Check sheet for the modelled part. Datum: model origin and axes. Units: mm. Face numbers are marked on the shaded views. A direction names the side the tool comes from. Give positions to 0.01 mm unless a question says otherwise; leave off trailing zeros. Loops run counter-clockwise (first coordinate to the right, second up) from the corner with the lowest first, then second, coordinate; pieces in that order, holes last. Notation, with made-up numbers: (38, -11) - (72, -11) arc R20 ccw to (72, 6) - close; hole circle Ø9 at (89, 33). An arc over 180 degrees is marked (long way). Use one line per item in the form item = value.
from build123d import *

# Parameters (mm, degrees)
CHANFREIN1_SIZE                     = 0.5
ENL_V_MAT_EXTRU_1_DEPTH             = 4
CHANFREIN2_SIZE                     = 1
DIAM_TRE_DU_PER_AGE_1_5_1_5_1_D     = 1.5
DIAM_TRE_DU_PER_AGE_1_5_1_5_1_DEPTH = 2
DIAM_TRE_DU_PER_AGE_1_5_1_5_1_TIP   = 0.450645464
CHANFREIN3_SIZE                     = 0.5
DIAM_TRE_DU_PER_AGE_1_5_1_5_2_D     = 1.5
DIAM_TRE_DU_PER_AGE_1_5_1_5_2_DEPTH = 2
DIAM_TRE_DU_PER_AGE_1_5_1_5_2_TIP   = 0.450645464
CHANFREIN4_SIZE                     = 0.5
BOSS_EXTRU_1_REACH                  = 77.975
ESQUISSE9_R                         = 7.5
ESQUISSE9_R_2                       = 4.5
CHANFREIN5_SIZE                     = 0.5


with BuildPart() as part:
    # Esquisse1 → Révolution1 (revolve)
    with BuildSketch(Plane.XY, mode=Mode.PRIVATE) as r_volution1_sk:
        Polygon((0, 0), (0, 5), (6, 5), (6, 4.75), (8, 4.75), (8, 7.5), (22, 7.5), (22, 13.6), (25, 13.6), (25, 9.75), (27, 9.75), (27, 10), (56, 10), (56, 8.5), (60, 8.5), (60, 5), (62, 5), (62, 6), (73.5, 6), (73.5, 0), align=None)
    revolve(r_volution1_sk.sketch.rotate(Axis((0, 0, 0), (1, 0, 0)), 90), axis=Axis((0, 0, 0), (1, 0, 0)))

    # Chanfrein1
    chanfrein1_edges = [part.edges().sort_by_distance(p)[0] for p in [
        (0, 0, -5),
        (8, 0, -4.75),
        (8, 0, -7.5),
        (25, 0, -13.6),
    ]]
    chamfer(chanfrein1_edges, length=CHANFREIN1_SIZE)

    # Esquisse2 → Enlèv. mat.-Extru.1 (cut)
    with BuildSketch(Plane(origin=(60, 0, 0), x_dir=(0, 0, -1), z_dir=(1, 0, 0))):
        with BuildLine():
            Line((-6, 12.573525265), (-6, -12.573525265))
            ThreePointArc((-6, -12.573525265), (-13.931745676, 0), (-6, 12.573525265))
        make_face()
        with BuildLine():
            Line((6, 12.573525265), (6, -12.573525265))
            ThreePointArc((6, -12.573525265), (13.931745676, 0), (6, 12.573525265))
        make_face()
    extrude(amount=-ENL_V_MAT_EXTRU_1_DEPTH, mode=Mode.SUBTRACT)

    # Chanfrein2
    chanfrein2_edges = [part.edges().sort_by_distance(p)[0] for p in [
        (73.5, 0, -6),
    ]]
    chamfer(chanfrein2_edges, length=CHANFREIN2_SIZE)

    # Diamètre du perçage Ø1.5 (1.5)1
    with Locations(Plane(origin=(73.5, 0, 0), x_dir=(0, 0, -1), z_dir=(1, 0, 0))):
        with Locations((0, 0)):
            Hole(DIAM_TRE_DU_PER_AGE_1_5_1_5_1_D / 2, depth=DIAM_TRE_DU_PER_AGE_1_5_1_5_1_DEPTH)
            with Locations((0, 0, -(DIAM_TRE_DU_PER_AGE_1_5_1_5_1_DEPTH + DIAM_TRE_DU_PER_AGE_1_5_1_5_1_TIP / 2))):  # 118° drill point
                Cone(0, DIAM_TRE_DU_PER_AGE_1_5_1_5_1_D / 2, DIAM_TRE_DU_PER_AGE_1_5_1_5_1_TIP, mode=Mode.SUBTRACT)

    # Chanfrein3
    chanfrein3_edges = [part.edges().sort_by_distance(p)[0] for p in [
        (73.5, 0, -0.75),
    ]]
    chamfer(chanfrein3_edges, length=CHANFREIN3_SIZE)

    # Diamètre du perçage Ø1.5 (1.5)2
    with Locations(Plane.ZY):
        with Locations((0, 0)):
            Hole(DIAM_TRE_DU_PER_AGE_1_5_1_5_2_D / 2, depth=DIAM_TRE_DU_PER_AGE_1_5_1_5_2_DEPTH)
            with Locations((0, 0, -(DIAM_TRE_DU_PER_AGE_1_5_1_5_2_DEPTH + DIAM_TRE_DU_PER_AGE_1_5_1_5_2_TIP / 2))):  # 118° drill point
                Cone(0, DIAM_TRE_DU_PER_AGE_1_5_1_5_2_D / 2, DIAM_TRE_DU_PER_AGE_1_5_1_5_2_TIP, mode=Mode.SUBTRACT)

    # Chanfrein4
    chanfrein4_edges = [part.edges().sort_by_distance(p)[0] for p in [
        (0, 0, 0.75),
    ]]
    chamfer(chanfrein4_edges, length=CHANFREIN4_SIZE)

    # Esquisse9 → Boss.-Extru.1 (add, up to next)
    with BuildSketch(Plane.ZY, mode=Mode.PRIVATE) as boss_extru_1_sk1:
        Circle(ESQUISSE9_R)
        Circle(ESQUISSE9_R_2, mode=Mode.SUBTRACT)
    boss_extru_1_tool1 = extrude(boss_extru_1_sk1.sketch, amount=-BOSS_EXTRU_1_REACH, mode=Mode.PRIVATE) - part.part
    add(boss_extru_1_tool1.solids().sort_by_distance((0, 0, -7.287868))[0])

    # Chanfrein5
    chanfrein5_edges = [part.edges().sort_by_distance(p)[0] for p in [
        (0, 0, -7.5),
    ]]
    chamfer(chanfrein5_edges, length=CHANFREIN5_SIZE)


solid = part.part
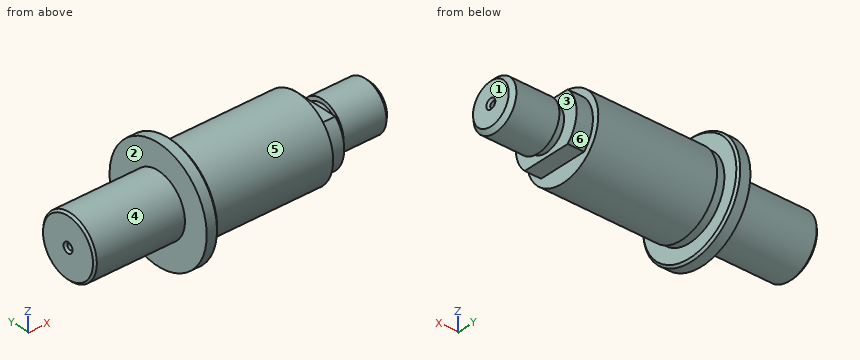
Item 1: Mould release check, pull along X, two halves, no side actions. Record for the marked faces 1, 2 and 3: released by +X, released by -X, zero draft, split by the parting line, or undercut.
Answer block:
face_1 = released by +X
face_2 = released by -X
face_3 = undercut
Item 2: Thickness scan on L1, parallel to Y at x = 72.3, z = 0; L2, parallel to Y at x = 1.6, z = 0; L3, parallel to X at y = 9.5, z = -6.5. Record the ranges inside material, lowest first.
Answer block:
L1 = -6 to -0.75, 0.75 to 6
L2 = -7.5 to -0.75, 0.75 to 7.5
L3 = 22 to 25
Item 3: Section check A-A on x = 28. Record the boundary of the cut face in (y, z), then the cut area to 3 significant figures.
Answer block:
outline = circle Ø20 at (0, 0)
area = 314 mm2
Item 4: Access from +Z, -Z, +X, -X, +Y, -Y to the whole of each face (thin tool, end or side, straight path). Record for the marked faces 4, 5 and 6.
Answer block:
face_4 = -X
face_5 = +X
face_6 = +X, +Y
Item 5: Gauge pin test, flat ends, axial feed: P1, Ø1, axis at x = 39, z = -5.5, coming from the -Y side; P2, Ø3, axis at x = 57, y = -2.5, coming from the -Z side; P3, Ø2, axis at x = 32, z = -7.5, coming from the +Y side; P4, Ø16, axis at y = 4, z = 3, coming from the -X side. Record the tip position at first contact, or that the pin passes through.
Answer block:
P1 = -8.66
P2 = -9.9
P3 = 7.6
P4 = 0
